```python
from build123d import *

# Parameters (mm, degrees)
BOSS_EXTRUDE1_DEPTH             = 2.6
SKETCH5_W                       = 11.826356456
SKETCH5_H                       = 5.621169426
CUT_EXTRUDE2_DEPTH              = 7.632050589
SKETCH6_W                       = 11.690711404
SKETCH6_H                       = 7.254613366
CUT_EXTRUDE3_DEPTH              = 5.2
SKETCH7_W                       = 0.5
SKETCH7_H                       = 0.5
BOSS_EXTRUDE2_DEPTH             = 12.7
BOSS_EXTRUDE2_DIRECTION_2_REACH = 8.542
SKETCH8_R                       = 0.8
CUT_EXTRUDE4_DEPTH              = 0.2


with BuildPart() as part:
    # Sketch2 → Boss-Extrude1 (new, symmetric)
    with BuildSketch(Plane(origin=(0, 0, 0), x_dir=(1, 0, 0), z_dir=(0, 1, 0))):
        with BuildLine():
            Line((-2.105447518, 1.212026432), (2.105447518, 1.212026432))
            ThreePointArc((2.105447518, 1.212026432), (0, -2.977973568), (-2.105447518, 1.212026432))
        make_face()
    extrude(amount=BOSS_EXTRUDE1_DEPTH, both=True)

    # Sketch5 → Cut-Extrude2 (cut, through all)
    with BuildSketch(Plane(origin=(0, 2.580250079, -0.225742631), x_dir=(1, 0, 0), z_dir=(0, 0.9961946980917455, -0.08715574274765836))):
        with Locations((0.924694538, -0.744658901)):
            Rectangle(SKETCH5_W, SKETCH5_H)
    cut_extrude2 = extrude(amount=CUT_EXTRUDE2_DEPTH, mode=Mode.SUBTRACT)

    # Sketch6 → Cut-Extrude3 (cut)
    with BuildSketch(Plane(origin=(0, 2.580250079, 0.225742631), x_dir=(1, 0, 0), z_dir=(0, 0.9961946980917467, 0.08715574274764504))):
        with Locations((0.257342704, -2.465539164)):
            Rectangle(SKETCH6_W, SKETCH6_H)
    cut_extrude3 = extrude(amount=CUT_EXTRUDE3_DEPTH, mode=Mode.SUBTRACT)

    # Mirror1: Cut-Extrude2, Cut-Extrude3 across plane
    add(cut_extrude2.mirror(Plane.ZX), mode=Mode.SUBTRACT)
    add(cut_extrude3.mirror(Plane.ZX), mode=Mode.SUBTRACT)


with BuildPart() as boss_extrude2_tool:
    # Sketch7 → Boss-Extrude2 (new body)
    with BuildSketch(Plane(origin=(0, -2.6, 0), x_dir=(-1, 0, 0), z_dir=(0, -1, 0))):
        with Locations((-1.27, 0.25)):
            Rectangle(SKETCH7_W, SKETCH7_H)
        with Locations((0, 0.25)):
            Rectangle(SKETCH7_W, SKETCH7_H)
        with Locations((1.27, 0.25)):
            Rectangle(SKETCH7_W, SKETCH7_H)
    extrude(amount=BOSS_EXTRUDE2_DEPTH)


with BuildPart() as part_1:
    add(part.part)


with BuildPart() as part_2:
    # Boss-Extrude2: joined with boss_extrude2_tool
    add(part_1.part.fuse(boss_extrude2_tool.part, tol=0.00001))

    # Sketch7 → Boss-Extrude2 direction 2 (add, up to next)
    with BuildSketch(Plane(origin=(0, -2.6, 0), x_dir=(-1, 0, 0), z_dir=(0, -1, 0)), mode=Mode.PRIVATE) as boss_extrude2_direction_2_sk1:
        with Locations((-1.27, 0.25)):
            Rectangle(SKETCH7_W, SKETCH7_H)
    boss_extrude2_direction_2_tool1 = extrude(boss_extrude2_direction_2_sk1.sketch, amount=-BOSS_EXTRUDE2_DIRECTION_2_REACH, mode=Mode.PRIVATE) - part_2.part
    # Sketch7 → Boss-Extrude2 direction 2 (add, up to next)
    with BuildSketch(Plane(origin=(0, -2.6, 0), x_dir=(-1, 0, 0), z_dir=(0, -1, 0)), mode=Mode.PRIVATE) as boss_extrude2_direction_2_sk2:
        with Locations((0, 0.25)):
            Rectangle(SKETCH7_W, SKETCH7_H)
    boss_extrude2_direction_2_tool2 = extrude(boss_extrude2_direction_2_sk2.sketch, amount=-BOSS_EXTRUDE2_DIRECTION_2_REACH, mode=Mode.PRIVATE) - part_2.part
    # Sketch7 → Boss-Extrude2 direction 2 (add, up to next)
    with BuildSketch(Plane(origin=(0, -2.6, 0), x_dir=(-1, 0, 0), z_dir=(0, -1, 0)), mode=Mode.PRIVATE) as boss_extrude2_direction_2_sk3:
        with Locations((1.27, 0.25)):
            Rectangle(SKETCH7_W, SKETCH7_H)
    boss_extrude2_direction_2_tool3 = extrude(boss_extrude2_direction_2_sk3.sketch, amount=-BOSS_EXTRUDE2_DIRECTION_2_REACH, mode=Mode.PRIVATE) - part_2.part
    add(boss_extrude2_direction_2_tool1.solids().sort_by_distance((1.27, -2.6, -0.25))[0])
    add(boss_extrude2_direction_2_tool2.solids().sort_by_distance((0, -2.6, -0.25))[0])
    add(boss_extrude2_direction_2_tool3.solids().sort_by_distance((-1.27, -2.6, -0.25))[0])

    # Sketch8 → Cut-Extrude4 (cut)
    with BuildSketch(Plane.XY.offset(2.977973568)):
        Circle(SKETCH8_R)
    extrude(amount=-CUT_EXTRUDE4_DEPTH, mode=Mode.SUBTRACT)


solid = part_2.part
```
The model under review builds one solid part; all positions refer to its coordinate system, in mm. Round coordinates to 2 decimals unless told otherwise and drop trailing zeros. Loops run counter-clockwise (first coordinate to the right, second up) from the corner with the lowest first, then second, coordinate; pieces in that order, holes last. Notation, with made-up numbers: (28, -9.75) -> (50, -9.75) arc R23 ccw to (50, 24.25) -> close; hole circle Ø6 at (26.25, 56). An arc over 180 degrees is marked (long way). Answer in a Markdown table with one row per item.
1) Consider section A-A, the plane y = -11.25. Write out the cut boundary in (x, z).
Taken from the geometry:
| item | result |
|---|---|
| outline | (-1.52, -0.5) -> (-1.02, -0.5) -> (-1.02, 0) -> (-1.52, 0) -> close; (-0.25, -0.5) -> (0.25, -0.5) -> (0.25, 0) -> (-0.25, 0) -> close; (1.02, -0.5) -> (1.52, -0.5) -> (1.52, 0) -> (1.02, 0) -> close |
2) Consider section C-C, the plane y = -1. Write out the cut boundary in (x, z), plus the area to 3 significant figures.
Taken from the geometry:
| item | result |
|---|---|
| outline | (-2.11, -1.21) -> (2.11, -1.21) arc R2.62 ccw (long way) to start |
| area | 18.5 mm² |
3) Wall thickness on line 1 along X through (y, z) = (-4.75, -0.05); line 2 along Z through (x, y) = (-0.1, 0.75); line 3 along Z through (x, y) = (-1.3, -7.75): over which ranges is each line inside the solid? List them lowest first.
Taken from the geometry:
| item | result |
|---|---|
| line 1 | x = -1.52 to -1.02, -0.25 to 0.25, 1.02 to 1.52 |
| line 2 | z = -1.21 to 2.78 |
| line 3 | z = -0.5 to 0 |
4) Consider section D-D, the plane z = -0.9. Write out the cut boundary in (x, y), plus the area to 3 significant figures.
Taken from the geometry:
| item | result |
|---|---|
| outline | (-2.3, -2.52) -> (2.3, -2.52) -> (2.3, 2.52) -> (-2.3, 2.52) -> close |
| area | 23.2 mm² |
5) Draft analysis for pull direction Y (two halves, no side actions). For faces 1 (the flat face through (-0.04, 2.5, 1.14)), 2 (the flat face through (0, 0, 2.778)), 3 (the flat face through (0, 0, -1.212)), 4 (the flat face through (-0.04, -2.5, 1.14)), state which applies: pulls with the +Y half, pulls with the -Y half, needs draft (parallel to the pull), parting line crosses it, or undercut.
Taken from the geometry:
| item | result |
|---|---|
| face 1 | pulls with the +Y half |
| face 2 | undercut |
| face 3 | needs draft |
| face 4 | pulls with the -Y half |
6) Consider section B-B, the plane x = 0. Write out the cut boundary in (y, z), plus the area to 3 significant figures.
Taken from the geometry:
| item | result |
|---|---|
| outline | (-15.3, -0.5) -> (-2.56, -0.5) -> (-2.49, -1.21) -> (2.49, -1.21) -> (2.6, 0) -> (2.34, 2.98) -> (0.8, 2.98) -> (0.8, 2.78) -> (-0.8, 2.78) -> (-0.8, 2.98) -> (-2.34, 2.98) -> (-2.6, 0) -> (-15.3, 0) -> close |
| area | 26.9 mm² |
7) For pin 1 Ø0.6 at (y, z) = (-8, -0.5) entering from -X; pin 2 Ø0.5 at (x, y) = (0.5, 0) entering from +Z; pin 3 Ø3 at (x, y) = (-2, -9) entering from -Z, all flat-tipped, find the tip position at first contact; note any pin that passes through.
Taken from the geometry:
| item | result |
|---|---|
| pin 1 | stops at x = -1.52 |
| pin 2 | stops at z = 2.78 |
| pin 3 | stops at z = -0.5 |
